Can you work these out from the model? Positions are in its coordinate system, mm. A direction names the side the tool comes from. Round coordinates to 2 decimals unless told otherwise and drop trailing zeros. Order: outer loops, then holes, each group sorted by start corner. A loop starts at its lowest first (then second) coordinate and runs counter-clockwise, first axis right, second up.
Q1. We'd pull the mould along X, two halves only. Please class faces 4 (the face through (-1.73, -30.41, -7.81)), 5 (the face through (-8, -29, -3.3)), 6 (the face through (1.172, 0.406, 8.923)): pulls with the +X half, pulls with the -X half, needs draft (parallel to the pull), parting line crosses it, or undercut.
Q2. For faces 1 (the face through (0, -29.5, 0)), 2 (the face through (-3.434, 38.754, 4.952)), 3 (the face through (4, 54, 0)), which set-ups out of +Z, -Z, +X, -X, +Y, -Y let a thin tool reach every point of the face, with its end or its side?
Q3. If I drill on line 1 (Z direction, x = -3, y = 38.6); line 2 (Z direction, x = 0, y = -30.4); line 3 (Y direction, x = -7, z = 4) (3 decimals), over which ranges is the centre line in solid material (lowest first)?
Q4. If we section it at B-B (y = -21): Please give me the cut outline in (x, z).
Q5. Will these pins go through, and if not, where does the flat tip stop? P1, Ø6, axis at y = -6.5, z = -1.5, coming from the +X side; P2, Ø0.6, axis at x = -2.5, z = 2.5, coming from the +Y side; P3, Ø2.5, axis at x = -3, z = 3, coming from the -Y side; P4, Ø1.5, axis at x = 5, y = -11.5, coming from the +Z side.
Q6. If we section it at A-A (y = 43.5): Please give me the cut outline in (x, z).
Autodesk Inventor part; units mm, degrees
ref_plane "YZ Plane" through (0, 0, 0) normal (1, 0, 0) x (0, 1, 0)
ref_plane "XZ Plane" through (0, 0, 0) normal (0, 1, 0) x (-1, 0, 0)
ref_plane "XY Plane" through (0, 0, 0) normal (0, 0, 1) x (1, 0, 0)
sketch "Sketch1" plane through (0, 0, 0) normal (0, 1, 0) x (-1, 0, 0)
  circle A0 centre (0, 0) radius 9
  dimension "d0" = 18
extrude "Extrusion1" add sketch "Sketch1" along normal mid plane 58
thread "Thread1"
sketch "Sketch2" plane through (0, -29, 0) normal (0, -1, 0) x (1, 0, 0)
  circle A0 centre (0, 0) radius 8.5
  dimension "d13" = 17
extrude "Extrusion2" add sketch "Sketch2" along normal blind 2.5
sketch "Sketch3" plane through (0, -31.5, 0) normal (0, -1, 0) x (1, 0, 0)
  circle A0 centre (0, 0) radius 8
  circle A1 centre (0, 0) radius 8.5
  dimension "d14" = 0.5
extrude "Extrusion3" cut sketch "Sketch3" against normal blind 2 contours A0
fillet "Fillet1" radius 0.2 1 edges at (-8, -31.5, 0)
fillet "Fillet2" radius 0.05 1 edges at (-8.5, -31.5, 0)
sketch "Sketch4" plane through (0, 29, 0) normal (0, 1, 0) x (1, 0, 0)
  circle A0 centre (0, 0) radius 8.75
  dimension "d15" = 17.5
extrude "Extrusion4" add sketch "Sketch4" along normal blind 8
sketch "Sketch5" plane through (0, 37, 0) normal (0, 1, 0) x (1, 0, 0)
  circle A0 centre (0, 0) radius 8.55
  circle A1 centre (0, 0) radius 8.75
  dimension "d18" = 0.2
extrude "Extrusion5" add sketch "Sketch5" along normal blind 2 contours A0
fillet "Fillet3" radius 0.5 1 edges at (-8.55, 39, 0)
sketch "Sketch6" plane through (0, 39, 0) normal (0, 1, 0) x (1, 0, 0)
  circle A0 centre (4, 0) radius 2.5
  point P0 (0, 0)
  dimension "d22" = 5
  dimension "d23" = 4
sketch3d "3D Sketch1"
  line L0 (4, 39, 0) -> (4, 54, 0)
  dimension "d26" = 15
sweep "Sweep2" add profiles "Sketch6" path "3D Sketch1"
sketch "Sketch7" plane through (0, 39, 0) normal (0, 1, 0) x (1, 0, 0)
  circle A0 centre (-3, -3) radius 2
  circle A1 centre (-3, -3) radius 1.45
  line L0 (-4.4283, -3.25) -> (-1.5717, -3.25)
  line L1 (-4.4283, -2.75) -> (-1.5717, -2.75)
  point P0 (0, 0)
  dimension "d29" = 4
  dimension "d30" = 3
  dimension "d31" = 3
  dimension "d32" = 2.9
  dimension "d33" = 0.5
  dimension "d34" = 0.25
extrude "Extrusion6" cut sketch "Sketch7" against normal blind 0.5
extrude "Extrusion7" cut sketch "Sketch7" against normal blind 0.3 contours A1 L0 L1
sketch "Sketch8" plane through (0, 39, 0) normal (0, 1, 0) x (1, 0, 0)
  circle A0 centre (-3, 4) radius 0.75
  point P0 (0, 0)
  dimension "d39" = 1.5
  dimension "d40" = 4
  dimension "d41" = 3
extrude "Extrusion8" add sketch "Sketch8" along normal blind 1
fillet "Fillet4" radius 0.75 1 edges at (-3.75, 40, -4)
sketch "Sketch9" plane through (0, -29.5, 0) normal (0, -1, 0) x (1, 0, 0)
  line L0 (1.5, 5) -> (-1.5, 5)
  line L1 (-1.5, 5) -> (-1.5, 1)
  line L2 (-1.5, 1) -> (1.5, 1)
  line L3 (1.5, 1) -> (1.5, 5)
  line L4 (1.5, -1) -> (-1.5, -1)
  line L5 (-1.5, -1) -> (-1.5, -5)
  line L6 (-1.5, -5) -> (1.5, -5)
  line L7 (1.5, -5) -> (1.5, -1)
  point P0 (0, 0)
  point P1 (0, 1)
  dimension "d45" = 4
  dimension "d46" = 4
  dimension "d47" = 3
  dimension "d48" = 2
  dimension "d49" = 1
sketch "Sketch10" plane through (0, 0, 0) normal (1, 0, 0) x (0, 1, 0)
  line L0 (-29.5, -5) -> (-29.5, -1)
  line L1 (-29.5, 1) -> (-29.5, 5)
  spline S0 degree 2 poles (-29.5, -1) (-31.582, -1.7446) (-29.5, -5) knots 0 0 0 1 1 1
  spline S1 degree 2 poles (-29.5, 1) (-31.5, 3) (-29.5, 5) knots 0 0 0 1 1 1
  line L2 (-29.5, -8) -> (-29.5, 8)
  point P0 (0, 0)
  point P1 (-30.5, -2)
  point P2 (-30.5, 3)
  dimension "d50" = 5
  dimension "d51" = 1
  dimension "d52" = 6
properties part number "2309HCMUTE-CDT23-CB_E3F-DS30C4" material "PVC-Piping"
Solution:
1. face 4: undercut
1. face 5: needs draft
1. face 6: parting line crosses it
2. face 1: -Y
2. face 2: +Y
2. face 3: +Z, -Z, +X, -X, +Y
3. line 1: z = -8 to 1, 1.55 to 4.45, 5 to 8
3. line 2: z = -8.5 to -8, 8 to 8.5
3. line 3: y = -31.445 to 39
4. outline: circle Ø18 at (0, 0)
5. P1: stops at x = 9
5. P2: stops at y = 39
5. P3: stops at y = -29.5
5. P4: stops at z = 7.93
6. outline: circle Ø5 at (4, 0)
